from build123d import *

# Parameters (mm, degrees)
SKETCH1_R           = 9.2
BOSS_EXTRUDE1_DEPTH = 3
SKETCH2_W           = 78.6
SKETCH2_H           = 3
BOSS_EXTRUDE2_DEPTH = 4


with BuildPart() as part:
    # Sketch1 → Boss-Extrude1 (new body)
    with BuildSketch(Plane(origin=(0, 0, 0), x_dir=(1, 0, 0), z_dir=(0, 1, 0))):
        with BuildLine():
            Line((0, 49), (58.2, 49))
            ThreePointArc((58.2, 49), (65.412489168, 46.012489168), (68.4, 38.8))
            Line((68.4, 38.8), (68.4, 0))
            Line((68.4, 0), (68.4, -12.2))
            Line((68.4, -12.2), (-10.2, -12.2))
            Line((-10.2, -12.2), (-10.2, 0))
            Line((-10.2, 0), (-10.2, 38.8))
            ThreePointArc((-10.2, 38.8), (-7.212489168, 46.012489168), (0, 49))
        make_face()
        with Locations(Location((0, 0, 0), (0, 0, 270))):
            Circle(SKETCH1_R, mode=Mode.SUBTRACT)
        with Locations(Location((19.4, 0, 0), (0, 0, 270))):
            Circle(SKETCH1_R, mode=Mode.SUBTRACT)
        with Locations(Location((38.8, 0, 0), (0, 0, 270))):
            Circle(SKETCH1_R, mode=Mode.SUBTRACT)
        with Locations(Location((58.2, 0, 0), (0, 0, 270))):
            Circle(SKETCH1_R, mode=Mode.SUBTRACT)
        with Locations(Location((19.4, 19.4, 0), (0, 0, 270))):
            Circle(SKETCH1_R, mode=Mode.SUBTRACT)
        with Locations(Location((38.8, 19.4, 0), (0, 0, 270))):
            Circle(SKETCH1_R, mode=Mode.SUBTRACT)
        with Locations(Location((58.2, 19.4, 0), (0, 0, 270))):
            Circle(SKETCH1_R, mode=Mode.SUBTRACT)
        with Locations(Location((19.4, 38.8, 0), (0, 0, 270))):
            Circle(SKETCH1_R, mode=Mode.SUBTRACT)
        with Locations(Location((38.8, 38.8, 0), (0, 0, 270))):
            Circle(SKETCH1_R, mode=Mode.SUBTRACT)
        with Locations(Location((58.2, 38.8, 0), (0, 0, 270))):
            Circle(SKETCH1_R, mode=Mode.SUBTRACT)
        with Locations(Location((0, 19.4, 0), (0, 0, 270))):
            Circle(SKETCH1_R, mode=Mode.SUBTRACT)
        with Locations(Location((0, 38.8, 0), (0, 0, 270))):
            Circle(SKETCH1_R, mode=Mode.SUBTRACT)
    extrude(amount=BOSS_EXTRUDE1_DEPTH)

    # Sketch2 → Boss-Extrude2 (add)
    with BuildSketch(Plane(origin=(0, 3, 0), x_dir=(1, 0, 0), z_dir=(0, 1, 0))):
        with Locations((29.1, -10.7)):
            Rectangle(SKETCH2_W, SKETCH2_H)
    extrude(amount=BOSS_EXTRUDE2_DEPTH)


solid = part.part
Check sheet for the modelled part. Datum: model origin and axes. Units: mm. A direction names the side the tool comes from. Round coordinates to 2 decimals unless told otherwise and drop trailing zeros. Loops run counter-clockwise (first coordinate to the right, second up) from the corner with the lowest first, then second, coordinate; pieces in that order, holes last. Notation, with made-up numbers: (61, -24) -> (74, -24) arc R25 cw to (74, -10) -> close; hole circle Ø8 at (0, 8). An arc over 180 degrees is marked (long way). Put each result on its own line as item: value. Start each with the question number.
1. Scan lines: probe 1 along X at (y, z) = (1.55, 0); probe 2 along Z at (x, y) = (20, 0.75); probe 3 along X at (y, z) = (1.5, -40.5). Record each from-to range of solid material in increasing order.
2. Access from +Z, -Z, +X, -X, +Y, -Y to the whole of each face (thin tool, end or side, straight path). Record for faces 1 (the face through (64.42, 1.48, -26.18)), 2 (the face through (29, 3, -20)).
3. Section check C-C (x = 62). Enter the section's corners in (y, z), plus the area to 3 significant figures.
4. Draft check along Z on faces 3 (the face through (29, 1, -49)), 4 (the face through (35.28, 1.48, -30.3)), 5 (the face through (29, 7, 11)). Enter one of: +Z half, -Z half, draft (parallel to the pull), parting line (faces both ways), or undercut.
5. Section check B-B (y = 1.5). Give the number of separate pieces and of enclosed holes in the cut face, plus the area to 3 significant figures.
6. Section check A-A (z = 0). Enter the section's corners in (x, y), plus the area to 3 significant figures.
7. Gauge pin test, flat ends, axial feed: pin 1 (14.5 mm diameter, centred on x = 19.4, z = -38.8, fed in from +Y); pin 2 (21 mm diameter, centred on x = 38.8, z = -19.4, fed in from +Y); pin 3 (1.2 mm diameter, centred on x = 24, y = 5.5, fed in from -Z). Record the tip position at first contact, or that the pin passes through.
8. Section check D-D (z = -27). Enter the section's corners in (x, y).
Findings:
1. probe 1: x = -10.2 to -9.2, 9.2 to 10.2, 28.6 to 29.6, 48 to 49, 67.4 to 68.4
1. probe 2: z = -49 to -47.98, -29.62 to -28.58, -10.22 to -9.18, 9.18 to 12.2
1. probe 3: x = -10.06 to -9.04, 9.04 to 10.36, 28.44 to 29.76, 47.84 to 49.16, 67.24 to 68.26
2. face 1: +Y, -Y
2. face 2: -Z, +X, -X, +Y
3. outline: (0, -48.27) -> (3, -48.27) -> (3, -47.18) -> (0, -47.18) -> close; (0, -30.42) -> (3, -30.42) -> (3, -27.78) -> (0, -27.78) -> close; (0, -11.02) -> (3, -11.02) -> (3, -8.38) -> (0, -8.38) -> close; (0, 8.38) -> (3, 8.38) -> (3, 9.2) -> (7, 9.2) -> (7, 12.2) -> (0, 12.2) -> close
3. area: 42.6 mm^2
4. face 3: -Z half
4. face 4: undercut
4. face 5: draft
5. separate pieces: 1
5. enclosed holes: 12
5. area: 1,570 mm^2
6. outline: (-10.2, 0) -> (-9.2, 0) -> (-9.2, 3) -> (-10.2, 3) -> close; (9.2, 0) -> (10.2, 0) -> (10.2, 3) -> (9.2, 3) -> close; (28.6, 0) -> (29.6, 0) -> (29.6, 3) -> (28.6, 3) -> close; (48, 0) -> (49, 0) -> (49, 3) -> (48, 3) -> close; (67.4, 0) -> (68.4, 0) -> (68.4, 3) -> (67.4, 3) -> close
6. area: 15.0 mm^2
7. pin 1: passes through
7. pin 2: stops at y = 3
7. pin 3: stops at z = 9.2
8. outline: (-10.2, 0) -> (-5.18, 0) -> (-5.18, 3) -> (-10.2, 3) -> close; (5.18, 0) -> (14.22, 0) -> (14.22, 3) -> (5.18, 3) -> close; (24.58, 0) -> (33.62, 0) -> (33.62, 3) -> (24.58, 3) -> close; (43.98, 0) -> (53.02, 0) -> (53.02, 3) -> (43.98, 3) -> close; (63.38, 0) -> (68.4, 0) -> (68.4, 3) -> (63.38, 3) -> close
